Read the model definition and answer for the solid it produces. Units are mm, in the model's axes. A direction names the side the tool comes from. Give positions to 0.01 mm unless a question says otherwise; leave off trailing zeros. Write each loop counter-clockwise with the first axis right and the second up, starting at its lowest first coordinate (ties: lowest second). Pieces come first, ordered by that corner, then holes. Notation, with made-up numbers: (70, -34.5) - (98, -34.5) arc R27 cw to (98, 0.5) - close; hole circle Ø9 at (-30, -9.75). An arc over 180 degrees is marked (long way). Answer as a JSON object with one key per item and string values. Group by question number.
```python
from build123d import *

# Parameters (mm, degrees)
SKETCH2_R                = 1.5
BOSS_EXTRUDE1_DEPTH      = 0.75
BOSS_EXTRUDE2_DEPTH      = 2.25
BOSS_EXTRUDE2_DEPTH_BACK = 0.75
SKETCH2_3_R              = 2.5
SKETCH2_3_R_2            = 1.25


with BuildPart() as part:
    # Sketch1 → Revolve1 (revolve)
    with BuildSketch(Plane.XY):
        with BuildLine():
            Line((0, 9), (0, -9))
            ThreePointArc((0, -9), (-9, 0), (0, 9))
        make_face()
    revolve(axis=Axis((0, 9, 0), (0, -1, 0)))

    # Sketch2 → Boss-Extrude1 (add, symmetric)
    with BuildSketch(Plane.XY):
        with BuildLine():
            Line((2.5, 8.645808233), (2.5, 46))
            ThreePointArc((2.5, 46), (0, 43.5), (-2.5, 46))
            Line((-2.5, 46), (-2.5, 8.645808233))
            Line((-2.5, 8.645808233), (-2.5, 6.974093444))
            Line((-2.5, 6.974093444), (2.5, 6.974093444))
            Line((2.5, 6.974093444), (2.5, 8.645808233))
        make_face()
        with Locations((0, 18)):
            Circle(SKETCH2_R, mode=Mode.SUBTRACT)
    extrude(amount=BOSS_EXTRUDE1_DEPTH, both=True)

    # Sketch2_3 → Boss-Extrude2 (add, two sides: drawn at the far end of the back side and taken through both)
    with BuildSketch(Plane.XY.offset(-BOSS_EXTRUDE2_DEPTH_BACK)):
        with Locations((0, 46)):
            Circle(SKETCH2_3_R)
        with Locations((0, 46)):
            Circle(SKETCH2_3_R_2, mode=Mode.SUBTRACT)
    extrude(amount=BOSS_EXTRUDE2_DEPTH + BOSS_EXTRUDE2_DEPTH_BACK)


solid = part.part
```
1) Find section C-C, the plane y = 32. Write down the section's boundary in (x, z), and give its area (3 significant figures).
2) Find section B-B, the plane y = 18. Write down the section's boundary in (x, z).
3) Flat-ended cylindrical pins translate along their axes: pin 1 Ø4 at (x, y) = (0.5, 19) entering from -Z; pin 2 Ø5 at (x, y) = (3.5, 3) entering from +Z; pin 3 Ø10 at (x, y) = (-4, 17) entering from +Z. Find the tip coordinate at first contact, or state that the pin passes through.
4) Find section A-A, the plane x = 0. Write down the section's boundary in (y, z).
5) For a pull along Y with two mould halves and no side action, classify faces 5 (the cylindrical face through (-0.16, 47.24, 0.73)), 6 (the flat face through (1, 47, 2.25)) as released by +Y, released by -Y, zero draft, split by the parting line, or undercut.
6) Find section D-D, the plane z = -3.5. Write down the section's boundary in (x, y), and give its area (3 significant figures).
7) Which of the six approach directions +Z, -Z, +X, -X, +Y, -Y give full straight-line access (tool end or side, diameter ignored) to faces 1 (the cylindrical face through (-0.33, 48.48, 1.06)), 2 (the flat face through (2.5, 27, 0)), 3 (the cylindrical face through (-0.195, 19.487, -0.01)), 4 (the flat face through (-2.5, 28, 0))?
8) Find the intervals of material crossed by line 1 (Y direction, x = 0, z = 0.1); line 2 (Y direction, x = 0, z = 1.5); line 3 (Z direction, x = 2, y = 9.5), in increasing order. Write a range as [from, to].
Values follow:
{
 "1": {"outline": "(-2.5, -0.75) - (2.5, -0.75) - (2.5, 0.75) - (-2.5, 0.75) - close", "area": "7.50 mm2"},
 "2": {"outline": "(-2.5, -0.75) - (-1.5, -0.75) - (-1.5, 0.75) - (-2.5, 0.75) - close; (1.5, -0.75) - (2.5, -0.75) - (2.5, 0.75) - (1.5, 0.75) - close"},
 "3": {"pin 1": "stops at z = -0.75", "pin 2": "stops at z = 8.75", "pin 3": "stops at z = 0.75"},
 "4": {"outline": "(8.97, -0.75) - (16.5, -0.75) - (16.5, 0.75) - (8.97, 0.75) arc R9 ccw (long way) to start; (19.5, -0.75) - (44.75, -0.75) - (44.75, 2.25) - (43.5, 2.25) - (43.5, 0.75) - (19.5, 0.75) - close; (47.25, -0.75) - (48.5, -0.75) - (48.5, 2.25) - (47.25, 2.25) - close"},
 "5": {"face 5": "undercut", "face 6": "zero draft"},
 "6": {"outline": "circle Ø16.58 at (0, 0)", "area": "216 mm2"},
 "7": {"face 1": "+Z", "face 2": "+Z, -Z, +X, +Y", "face 3": "+Z, -Z", "face 4": "+Z, -Z, -X, +Y"},
 "8": {"line 1": "y = [-9, 16.5], [19.5, 44.75], [47.25, 48.5]", "line 2": "y = [-8.87, 8.87], [43.5, 44.75], [47.25, 48.5]", "line 3": "z = [-0.75, 0.75]"}
}
